Verification items for the finished model (mm, model axes). Round coordinates to 2 decimals unless told otherwise and drop trailing zeros. Write each loop counter-clockwise with the first axis right and the second up, starting at its lowest first coordinate (ties: lowest second). Pieces come first, ordered by that corner, then holes. Notation, with made-up numbers: M 21,77.25 L 79,77.25 A16 cw 79,94.25 Z; hole C 63.5,49 d5. An arc over 180 degrees is marked long. One line per question, with ' | ' between items.
from build123d import *

# Parameters (mm, degrees)
SKETCH_1_W          = 23.2
SKETCH_1_H          = 22.5
EXTRUDE_1_DEPTH     = 1.5
FILLET_1_R          = 2
SKETCH_2_R          = 1.8
CUT_EXTRUDE_1_DEPTH = 1.5
SKETCH_3_W          = 3.6
SKETCH_3_H          = 4.9
EXTRUDE_2_DEPTH     = 1.5
CHAMFER_1_SIZE      = 0.2
SKETCH_17_R         = 0.5
CUT_EXTRUDE_2_DEPTH = 0.1


with BuildPart() as part:
    # 草图1 → 凸台-拉伸1 (new body)
    with BuildSketch(Plane(origin=(0, 0, 0), x_dir=(1, 0, 0), z_dir=(0, 1, 0))):
        Rectangle(SKETCH_1_W, SKETCH_1_H)
    extrude(amount=EXTRUDE_1_DEPTH)

    # 圆角1
    fillet_1_edges = [part.edges().sort_by_distance(p)[0] for p in [
        (11.6, 0.75, 11.25),
        (-11.6, 0.75, 11.25),
        (-11.6, 0.75, -11.25),
        (11.6, 0.75, -11.25),
    ]]
    fillet(fillet_1_edges, radius=FILLET_1_R)

    # 草图2 → 切除-拉伸1 (cut)
    with BuildSketch(Plane.XZ):
        with Locations(Location((-8, 8, 0), (0, 0, 270))):
            Circle(SKETCH_2_R)
        with Locations(Location((8, 8, 0), (0, 0, 270))):
            Circle(SKETCH_2_R)
        with Locations(Location((8, -8, 0), (0, 0, 270))):
            Circle(SKETCH_2_R)
        with Locations(Location((-8, -8, 0), (0, 0, 270))):
            Circle(SKETCH_2_R)
    extrude(amount=-CUT_EXTRUDE_1_DEPTH, mode=Mode.SUBTRACT)

    # 草图3 → 凸台-拉伸2 (add)
    with BuildSketch(Plane(origin=(0, 1.5, 0), x_dir=(1, 0, 0), z_dir=(0, 1, 0))):
        Rectangle(SKETCH_3_W, SKETCH_3_H)
    extrude(amount=EXTRUDE_2_DEPTH)

    # 倒角1
    chamfer_1_edges = [part.edges().sort_by_distance(p)[0] for p in [
        (1.8, 3, 0),
        (-1.8, 3, 0),
    ]]
    chamfer(chamfer_1_edges, length=CHAMFER_1_SIZE)

    # 草图17 → 切除-拉伸2 (cut)
    with BuildSketch(Plane.XZ):
        with Locations(Location((0, 0, 0), (0, 0, 270))):
            Circle(SKETCH_17_R)
    extrude(amount=-CUT_EXTRUDE_2_DEPTH, mode=Mode.SUBTRACT)


solid = part.part
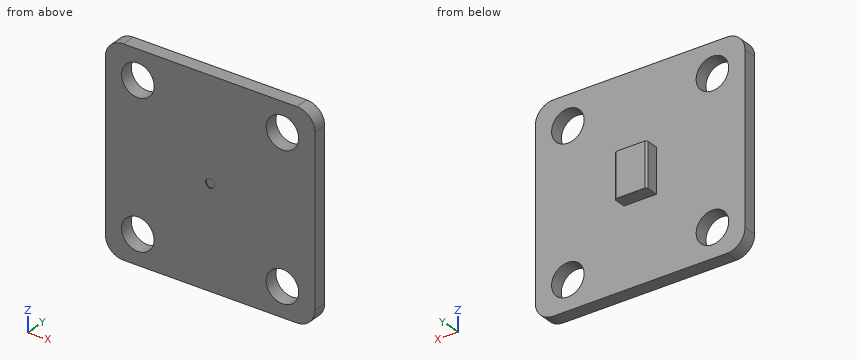
1. Go/stop test with flat-tipped pins: P1, Ø0.5, axis at x = -0.5, y = 2.5, coming from the +Z side; P2, Ø0.5, axis at x = 0, z = 0, coming from the -Y side; P3, Ø3, axis at x = -8, z = 8, coming from the -Y side; P4, Ø4.5, axis at x = 8, z = -8, coming from the +Y side. Record where each tip stops, or that it passes through.
Results:
P1: stops at z = 2.45 | P2: stops at y = 0.1 | P3: passes through | P4: stops at y = 1.5
2. Thickness scan on line 1 (X direction, y = 0.9, z = -8); line 2 (Y direction, x = 10.5, z = -4); line 3 (Z direction, x = -9, y = 1.4). Record the ranges inside material, lowest first.
Results:
line 1: x = -11.6 to -9.8, -6.2 to 6.2, 9.8 to 11.6 | line 2: y = 0 to 1.5 | line 3: z = -11.25 to -9.5, -6.5 to 6.5, 9.5 to 11.25
3. Section check C-C, the plane y = 1. Record the cut outline in (x, z), then the cut area to 3 significant figures.
Results:
outline: M -11.6,-9.25 A2 ccw -9.6,-11.25 L 9.6,-11.25 A2 ccw 11.6,-9.25 L 11.6,9.25 A2 ccw 9.6,11.25 L -9.6,11.25 A2 ccw -11.6,9.25 Z; hole C -8,-8 d3.6; hole C -8,8 d3.6; hole C 8,-8 d3.6; hole C 8,8 d3.6 | area: 478 mm2
4. Section check D-D, the plane z = -2. Record the cut outline in (x, y).
Results:
outline: M -11.6,0 L 11.6,0 L 11.6,1.5 L 1.8,1.5 L 1.8,2.8 L 1.6,3 L -1.6,3 L -1.8,2.8 L -1.8,1.5 L -11.6,1.5 Z
5. Section check A-A, the plane z = -8. Record the cut outline in (x, y), then the cut area to 3 significant figures.
Results:
outline: M -11.6,0 L -9.8,0 L -9.8,1.5 L -11.6,1.5 Z; M -6.2,0 L 6.2,0 L 6.2,1.5 L -6.2,1.5 Z; M 9.8,0 L 11.6,0 L 11.6,1.5 L 9.8,1.5 Z | area: 24.0 mm2
6. Section check B-B, the plane x = -8. Record the cut outline in (y, z), then the cut area to 4 significant figures.
Results:
outline: M 0,-11.25 L 1.5,-11.25 L 1.5,-9.8 L 0,-9.8 Z; M 0,-6.2 L 1.5,-6.2 L 1.5,6.2 L 0,6.2 Z; M 0,9.8 L 1.5,9.8 L 1.5,11.25 L 0,11.25 Z | area: 22.95 mm2
